Check sheet for the drawn part. Datum: minimum x, y, z corner. Units: mm. A direction names the side the tool comes from. Give positions to 0.01 mm unless a question says otherwise; leave off trailing zeros. Loops run counter-clockwise (first coordinate to the right, second up) from the corner with the lowest first, then second, coordinate; pieces in that order, holes last. Notation, with made-up numbers: M 27.25,62.5 L 70.25,62.5 A30 cw 70.25,97.5 Z; hole C 85,43.5 d2. An arc over 180 degrees is marked long. Write each question's results on one line, items separated by ' | '. Start each with the question number.
1. Material ranges on line 1 along Z through (x, y) = (2.7, 5); line 2 along Z through (x, y) = (5.25, 16.75); line 3 along Z through (x, y) = (2.45, 4.5), recorded low to high.
2. Sectioned sample at D-D on y = 14.75. Record the cut outline in (x, z), and give its area (3 significant figures).
3. Tool access check on the marked faces 1, 2, 3 and 4. Record the directions out of +Z, -Z, +X, -X, +Y, -Y that give a thin tool (end or side, any length) a straight path to the whole face; none if there is none.
4. Draft check along Z on the marked faces 5, 6, 7 and 8. Enter one of: pulls with the +Z half, pulls with the -Z half, needs draft (parallel to the pull), parting line crosses it, or undercut.
5. Sectioned sample at A-A on z = 27.5. Record the cut outline in (x, y).
6. Sectioned sample at B-B on y = 5. Record the cut outline in (x, z), and give its area (3 significant figures).
7. Go/stop test with a flat-tipped pin: pin 1 (3 mm diameter, centred on x = 4, z = 18, fed in from +Y). Record where the tip stops, or that it passes through.
8. Sectioned sample at C-C on x = 3.5. Record the cut outline in (y, z), and give its area (3 significant figures).
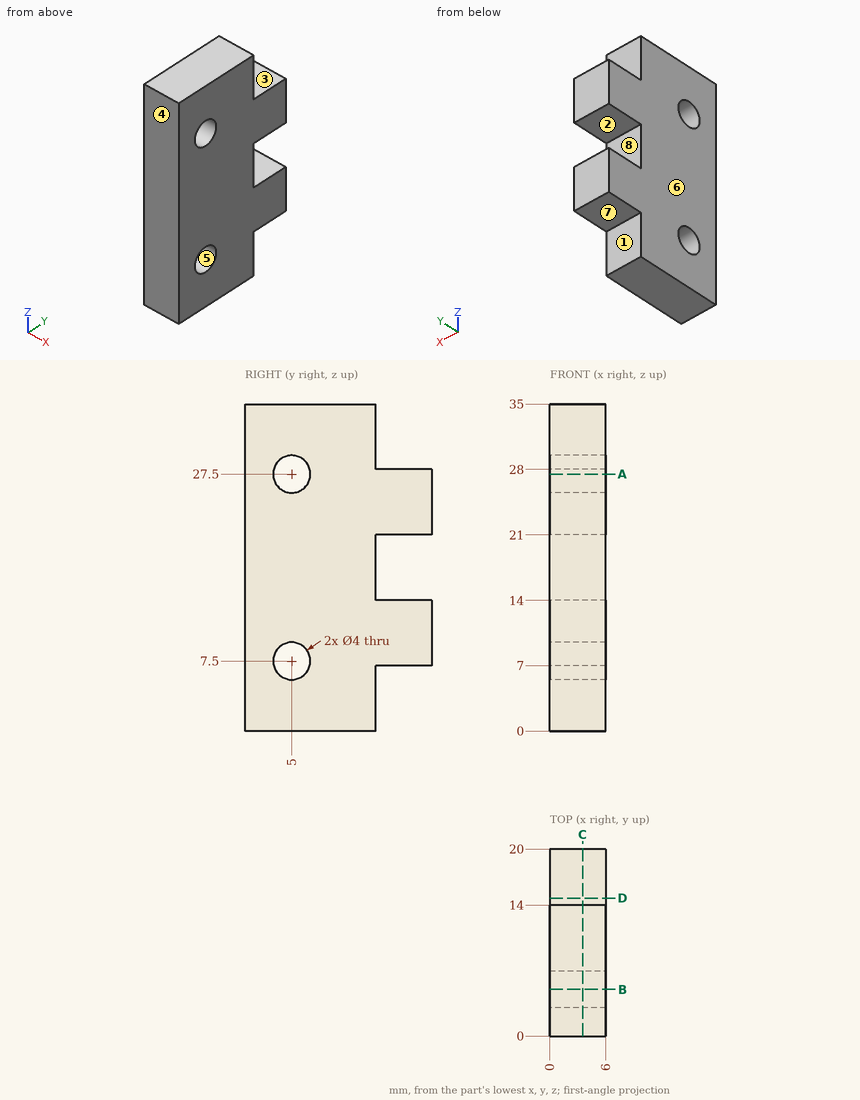
Output values:
1) line 1: 0 to 5.5, 9.5 to 25.5, 29.5 to 35 | line 2: 7 to 14, 21 to 28 | line 3: 0 to 5.56, 9.44 to 25.56, 29.44 to 35
2) outline: M 0,7 L 6,7 L 6,14 L 0,14 Z; M 0,21 L 6,21 L 6,28 L 0,28 Z | area: 84.0 mm2
3) face 1: -Z, +X, -X, +Y | face 2: +X, -X, +Y | face 3: +Z, +X, -X, +Y | face 4: +Z, -Z, +X, -X, -Y
4) face 5: undercut | face 6: needs draft | face 7: pulls with the -Z half | face 8: undercut
5) outline: M 0,0 L 6,0 L 6,3 L 0,3 Z; M 0,7 L 6,7 L 6,20 L 0,20 Z
6) outline: M 0,0 L 6,0 L 6,5.5 L 0,5.5 Z; M 0,9.5 L 6,9.5 L 6,25.5 L 0,25.5 Z; M 0,29.5 L 6,29.5 L 6,35 L 0,35 Z | area: 162 mm2
7) pin 1: y = 14
8) outline: M 0,0 L 14,0 L 14,7 L 20,7 L 20,14 L 14,14 L 14,21 L 20,21 L 20,28 L 14,28 L 14,35 L 0,35 Z; hole C 5,7.5 d4; hole C 5,27.5 d4 | area: 549 mm2
